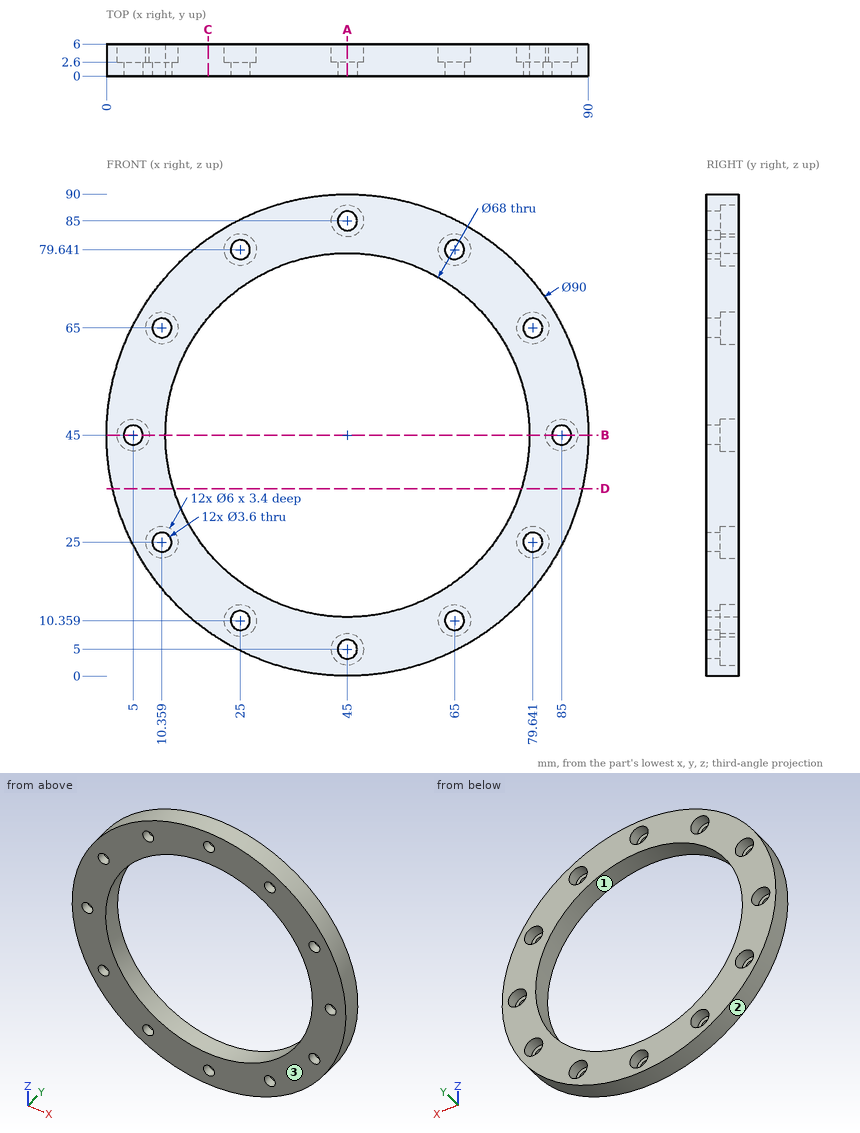
The drawing under review shows one solid part. Ordinate dimensions are in mm from its lowest x, y, z. Coordinates: 2 decimals unless noted, no trailing zeros. Write each loop counter-clockwise with the first axis right and the second up, starting at its lowest first coordinate (ties: lowest second). Pieces come first, ordered by that corner, then holes. Notation, with made-up numbers: (-7.5, 46) -> (47.5, 46) arc R36 cw to (47.5, 82) -> close; hole circle Ø3 at (-25.5, 27). An arc over 180 degrees is marked (long way). Write each question's results on one line, items separated by ' | '. Start each with the question number.
1) Consider section D-D (z = 35). Write out the cut boundary in (x, y).
2) Consider section C-C (x = 19). Write out the cut boundary in (y, z), plus the area to 3 significant figures.
3) Consider section B-B (z = 45). Write out the cut boundary in (x, y), plus the area to 3 significant figures.
4) Insertion check: pin 1 (1.8 mm diameter, centred on x = 66, z = 9, fed in from +Y); pin 2 (1 mm diameter, centred on y = 1, z = 44, fed in from -X); pin 3 (2 mm diameter, centred on x = 24, y = 0.5, fed in from +Z). Each pin has a flat end and moves straight along its axis. Give the tip position at first contact, or say it passes through.
5) Consider section A-A (x = 45). Write out the cut boundary in (y, z).
6) The part is to be moulded in two halves that separate along X. For the marked faces 1, 2 and 3, say which applies: +X half, -X half, draft (parallel to the pull), parting line (faces both ways), or undercut.
7) Wall thickness on L1, parallel to X at y = 1.7, z = 25; L2, parallel to X at y = 4.4, z = 44.5; L3, parallel to Z at x = 57, y = 1.5: over which ranges is each line inside the solid? List them lowest first. Write a range as [from, to].
Geometry says:
1) outline: (1.13, 0) -> (12.5, 0) -> (12.5, 6) -> (1.13, 6) -> close; (77.5, 0) -> (88.87, 0) -> (88.87, 6) -> (77.5, 6) -> close
2) outline: (0, 8.27) -> (6, 8.27) -> (6, 23.09) -> (0, 23.09) -> close; (0, 66.91) -> (6, 66.91) -> (6, 81.73) -> (0, 81.73) -> close | area: 178 mm^2
3) outline: (0, 0) -> (3.2, 0) -> (3.2, 2.6) -> (2, 2.6) -> (2, 6) -> (0, 6) -> close; (6.8, 0) -> (11, 0) -> (11, 6) -> (8, 6) -> (8, 2.6) -> (6.8, 2.6) -> close; (79, 0) -> (83.2, 0) -> (83.2, 2.6) -> (82, 2.6) -> (82, 6) -> (79, 6) -> close; (86.8, 0) -> (90, 0) -> (90, 6) -> (88, 6) -> (88, 2.6) -> (86.8, 2.6) -> close | area: 72.5 mm^2
4) pin 1: y = 2.6 | pin 2: x = 0 | pin 3: z = 85.31
5) outline: (0, 0) -> (6, 0) -> (6, 2) -> (2.6, 2) -> (2.6, 3.2) -> (0, 3.2) -> close; (0, 6.8) -> (2.6, 6.8) -> (2.6, 8) -> (6, 8) -> (6, 11) -> (0, 11) -> close; (0, 79) -> (6, 79) -> (6, 82) -> (2.6, 82) -> (2.6, 83.2) -> (0, 83.2) -> close; (0, 86.8) -> (2.6, 86.8) -> (2.6, 88) -> (6, 88) -> (6, 90) -> (0, 90) -> close
6) face 1: undercut | face 2: parting line | face 3: draft
7) L1: [4.69, 8.56], [12.16, 17.5], [72.5, 77.84], [81.44, 85.31] | L2: [0, 2.04], [7.96, 11], [79, 82.04], [87.96, 90] | L3: [1.63, 13.19], [76.81, 88.37]
